```python
from build123d import *

# Parameters (mm, degrees)
SKETCH1_W           = 5
SKETCH1_H           = 5
BOSS_EXTRUDE1_DEPTH = 10
BOSS_EXTRUDE2_DEPTH = 5
BOSS_EXTRUDE3_DEPTH = 5
SKETCH4_R           = 5
BOSS_EXTRUDE4_DEPTH = 5
SKETCH5_R           = 4
BOSS_EXTRUDE5_DEPTH = 80
SKETCH6_W           = 4
SKETCH6_H           = 4
CUT_EXTRUDE1_DEPTH  = 4


with BuildPart() as part:
    # Sketch1 → Boss-Extrude1 (new body)
    with BuildSketch(Plane(origin=(0, 0, 0), x_dir=(1, 0, 0), z_dir=(0, 1, 0))):
        Rectangle(SKETCH1_W, SKETCH1_H)
    extrude(amount=BOSS_EXTRUDE1_DEPTH)

    # Sketch2 → Boss-Extrude2 (add)
    with BuildSketch(Plane.XZ):
        Polygon((0, 7.5), (-6.495190528, 3.75), (-6.495190528, -3.75), (0, -7.5), (6.495190528, -3.75), (6.495190528, 3.75), align=None)
    extrude(amount=BOSS_EXTRUDE2_DEPTH)

    # Sketch3 → Boss-Extrude3 (add)
    with BuildSketch(Plane(origin=(0, 10, 0), x_dir=(1, 0, 0), z_dir=(0, 1, 0))):
        Polygon((0, -7.5), (6.495190528, -3.75), (6.495190528, 3.75), (0, 7.5), (-6.495190528, 3.75), (-6.495190528, -3.75), align=None)
    extrude(amount=BOSS_EXTRUDE3_DEPTH)

    # Sketch4 → Boss-Extrude4 (add)
    with BuildSketch(Plane(origin=(0, 15, 0), x_dir=(1, 0, 0), z_dir=(0, 1, 0))):
        Circle(SKETCH4_R)
    extrude(amount=BOSS_EXTRUDE4_DEPTH)

    # Sketch5 → Boss-Extrude5 (add)
    with BuildSketch(Plane(origin=(0, 20, 0), x_dir=(1, 0, 0), z_dir=(0, 1, 0))):
        Circle(SKETCH5_R)
    extrude(amount=BOSS_EXTRUDE5_DEPTH)

    # Sketch6 → Cut-Extrude1 (cut)
    with BuildSketch(Plane(origin=(0, 100, 0), x_dir=(1, 0, 0), z_dir=(0, 1, 0))):
        Rectangle(SKETCH6_W, SKETCH6_H)
    extrude(amount=-CUT_EXTRUDE1_DEPTH, mode=Mode.SUBTRACT)


solid = part.part
```
Could you check a few things on this model? Use its own coordinates, in mm. A direction names the side the tool comes from. Round coordinates to 2 decimals unless told otherwise and drop trailing zeros. Order: outer loops, then holes, each group sorted by start corner. A loop starts at its lowest first (then second) coordinate and runs counter-clockwise, first axis right, second up. Notation, with made-up numbers: M 74,66.25 L 95,66.25 A20 cw 95,91.25 Z; hole C 57,-2 d7. An arc over 180 degrees is marked long. One line per question, with ' | ' between items. Start each with the question number.
(1) For faces 4 (the face through (0, 10, 3)), 5 (the face through (-5, 15, -2)), 6 (the face through (0, 5, -2.5)), 7 (the face through (2.5, 5, 0)), which set-ups out of +Z, -Z, +X, -X, +Y, -Y let a thin tool reach every point of the face, with its end or its side?
(2) Thinking about a two-plate mould opening in Y: for faces 1 (the face through (0, 96, 0)), 2 (the face through (0, 0, -3)), 3 (the face through (-2, 98, 0)), which applies, +Y half, -Y half, draft (parallel to the pull), parting line (faces both ways), or undercut?
(3) Please list where these lines run through material, in increasing order: line 1 along Y through (x, z) = (-0.75, -5); line 2 along Y through (x, z) = (1.5, -4.25); line 3 along Z through (x, y) = (-0.25, 81.5).
(4) Suppose I cut it at B-B on y = 32. List the corners of the cut face in (x, z) for me, then the cut area to 3 significant figures.
(5) Suppose I cut it at A-A on z = 0. List the corners of the cut face in (x, y) for me, then the cut area to 3 significant figures.
(6) For P1, Ø1.2, axis at x = -0.5, z = 0.5, coming from the +Y side; P2, Ø5.5, axis at y = 4.5, z = 1, coming from the -X side; P3, Ø6, axis at x = 1.5, y = 57.5, coming from the +Z side, each with a flat end and sliding along its axis, tell me the tip position at first contact or that it passes through.
Geometry results:
1) face 4: none | face 5: +Y | face 6: -Z, +X, -X | face 7: +Z, -Z, +X
2) face 1: +Y half | face 2: undercut | face 3: draft
3) line 1: -5 to 0, 10 to 15 | line 2: -5 to 0, 10 to 20 | line 3: -3.99 to 3.99
4) outline: C 0,0 d8 | area: 50.3 mm²
5) outline: M -6.5,-5 L 6.5,-5 L 6.5,0 L 2.5,0 L 2.5,10 L 6.5,10 L 6.5,15 L 5,15 L 5,20 L 4,20 L 4,100 L 2,100 L 2,96 L -2,96 L -2,100 L -4,100 L -4,20 L -5,20 L -5,15 L -6.5,15 L -6.5,10 L -2.5,10 L -2.5,0 L -6.5,0 Z | area: 854 mm²
6) P1: y = 96 | P2: x = -2.5 | P3: z = 4
